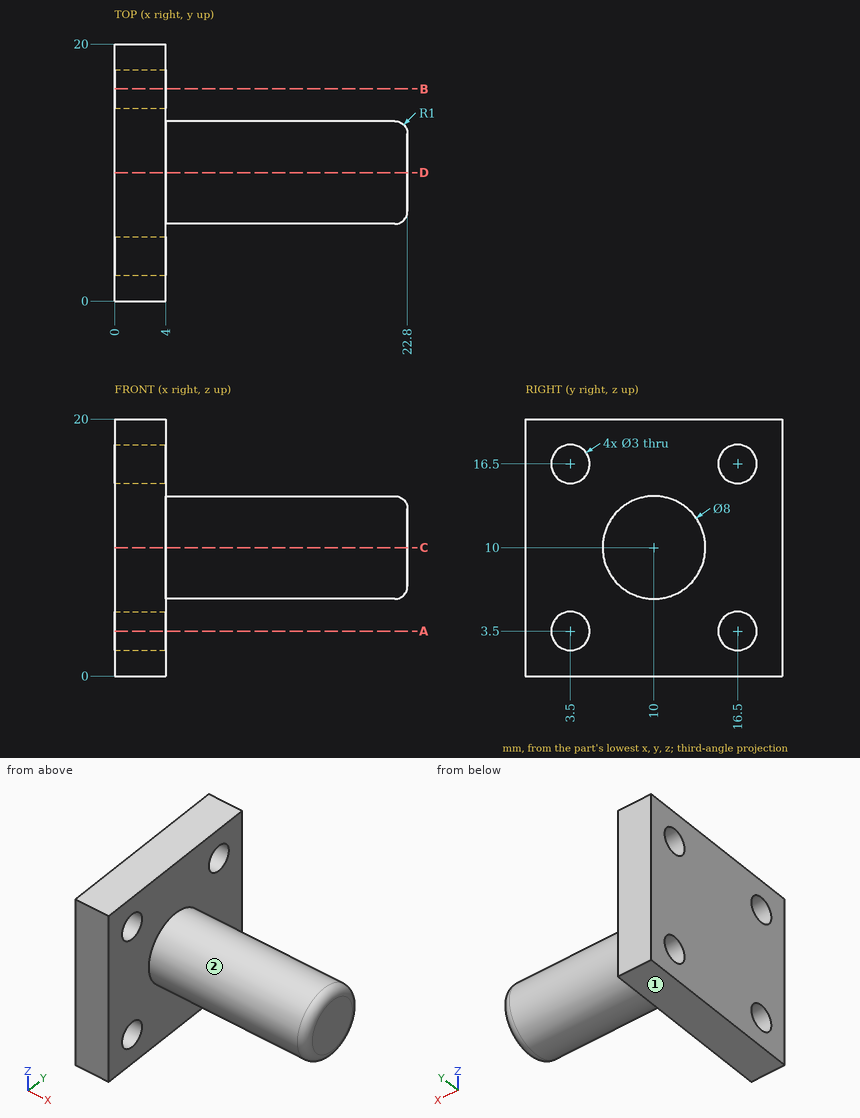
Verification items for this drawing (mm, ordinates from the low corner). A direction names the side the tool comes from. Coordinates: 2 decimals unless noted, no trailing zeros. Write each loop counter-clockwise with the first axis right and the second up, starting at its lowest first coordinate (ties: lowest second). Pieces come first, ordered by that corner, then holes. Notation, with made-up numbers: M 55.5,-38.5 L 71.5,-38.5 A24 ccw 71.5,-1.5 Z; hole C -10.75,-6.75 d4. An arc over 180 degrees is marked long. One line per item, written item: value. Start each with the question number.
(1) Sectioned sample at A-A, the plane z = 3.5. Enter the section's corners in (x, y).
(2) Scan lines: line 1 along Y through (x, z) = (1.7, 16.5); line 2 along X through (y, z) = (4.25, 8.5); line 3 along Y through (x, z) = (8.75, 8). Record each from-to range of solid material in increasing order. Write a range as [from, to].
(3) Sectioned sample at C-C, the plane z = 10. Enter the section's corners in (x, y).
(4) Tool access check on the marked faces 1 and 2. Record the directions out of +Z, -Z, +X, -X, +Y, -Y that give a thin tool (end or side, any length) a straight path to the whole face; none if there is none.
(5) Depth check by flat-ended pin: pin 1 (8 mm diameter, centred on y = 16, z = 11, fed in from -X); pin 2 (8 mm diameter, centred on y = 5.5, z = 2.5, fed in from +X); pin 3 (2 mm diameter, centred on x = 10, y = 12.5, fed in from +Z); pin 4 (1 mm diameter, centred on x = 17, z = 13.5, fed in from +Y). Enter the tip coordinate at first touch or a pass-through.
Filled sheet:
1. outline: M 0,0 L 4,0 L 4,2 L 0,2 Z; M 0,5 L 4,5 L 4,15 L 0,15 Z; M 0,18 L 4,18 L 4,20 L 0,20 Z
2. line 1: [0, 2], [5, 15], [18, 20]
2. line 2: [0, 4]
2. line 3: [6.54, 13.46]
3. outline: M 0,0 L 4,0 L 4,6 L 21.8,6 A1 ccw 22.8,7 L 22.8,13 A1 ccw 21.8,14 L 4,14 L 4,20 L 0,20 Z
4. face 1: -Z, +X, -X, +Y, -Y
4. face 2: +X
5. pin 1: x = 0
5. pin 2: x = 4
5. pin 3: z = 13.71
5. pin 4: y = 12.65
